from build123d import *

# Parameters (mm, degrees)
SKETCH1_W           = 165.1
SKETCH1_H           = 127
BOSS_EXTRUDE1_DEPTH = 6.35
SKETCH2_W           = 165.1
SKETCH2_H           = 31.75
BOSS_EXTRUDE2_DEPTH = 31.75
CUT_EXTRUDE1_REACH  = 167.1
SKETCH3_R           = 9.525


with BuildPart() as part:
    # Sketch1 → Boss-Extrude1 (new body, symmetric)
    with BuildSketch(Plane(origin=(0, 0, 0), x_dir=(1, 0, 0), z_dir=(0, 1, 0))):
        Rectangle(SKETCH1_W, SKETCH1_H)
    extrude(amount=BOSS_EXTRUDE1_DEPTH, both=True)

    # Sketch2 → Boss-Extrude2 (add)
    with BuildSketch(Plane.XZ.offset(6.35)):
        Rectangle(SKETCH2_W, SKETCH2_H)
    extrude(amount=BOSS_EXTRUDE2_DEPTH)

    # Sketch3 → Cut-Extrude1 (cut, up to next)
    with BuildSketch(Plane(origin=(82.55, 0, 0), x_dir=(0, 0, -1), z_dir=(1, 0, 0)), mode=Mode.PRIVATE) as cut_extrude1_sk1:
        with Locations((0, -22.225)):
            Circle(SKETCH3_R)
    cut_extrude1_tool1 = extrude(cut_extrude1_sk1.sketch, amount=-CUT_EXTRUDE1_REACH, mode=Mode.PRIVATE) & part.part
    add(cut_extrude1_tool1.solids().sort_by_distance((82.55, -22.225, 0))[0], mode=Mode.SUBTRACT)


solid = part.part
The model under review builds one solid part; all positions refer to its coordinate system, in mm. A direction names the side the tool comes from. Round coordinates to 2 decimals unless told otherwise and drop trailing zeros. Order: outer loops, then holes, each group sorted by start corner. A loop starts at its lowest first (then second) coordinate and runs counter-clockwise, first axis right, second up. Notation, with made-up numbers: (34.5, -10.5) - (56.5, -10.5) arc R29 ccw to (56.5, 15.5) - close; hole circle Ø10 at (-34, 52.5). An arc over 180 degrees is marked (long way). Use one line per item in the form item = value.
Q1. Add section D-D on z = -44. Give the boundary of the cut face in (x, y), then the cut area to 3 significant figures.
Response values:
outline = (-82.55, -6.35) - (82.55, -6.35) - (82.55, 6.35) - (-82.55, 6.35) - close
area = 2,100 mm^2
Q2. Add section B-B on y = -24.5. Give the boundary of the cut face in (x, z) (3 decimals), then the cut area to 3 significant figures.
Response values:
outline = (-82.55, -15.875) - (82.55, -15.875) - (82.55, -9.249) - (-82.55, -9.249) - close; (-82.55, 9.249) - (82.55, 9.249) - (82.55, 15.875) - (-82.55, 15.875) - close
area = 2,190 mm^2
Q3. To check wall thickness, follow line 1 (Y direction, x = 41, z = 0); line 2 (Y direction, x = 2.5, z = 43); line 3 (Z direction, x = -41, y = -19) (3 decimals). State the ranges of each line that lie inside material, in increasing order.
Response values:
line_1 = -38.1 to -31.75, -12.7 to 6.35
line_2 = -6.35 to 6.35
line_3 = -15.875 to -8.962, 8.962 to 15.875
Q4. Tool access review of faces 1 (the flat face through (-1, -22, -15.875)), 2 (the flat face through (-1, -22, 15.875)), 3 (the flat face through (82.55, -11, 1)): name each direction out of +Z, -Z, +X, -X, +Y, -Y from which nothing blocks a thin tool from reaching the whole face with its end or side.
Response values:
face_1 = -Z, +X, -X, -Y
face_2 = +Z, +X, -X, -Y
face_3 = +Z, -Z, +X, +Y, -Y
Q5. Mouldability with a two-part tool opening along Y and no side actions: class faces 4 (the flat face through (-82.55, -11, 1)), 5 (the cylindrical face through (1.16, -12.78, 1.24)), 6 (the flat face through (-1, -6.35, 39)) as pulls with the +Y half, pulls with the -Y half, needs draft (parallel to the pull), parting line crosses it, or undercut.
Response values:
face_4 = needs draft
face_5 = undercut
face_6 = pulls with the -Y half
Q6. Clearance check with flat-ended pins moving along their axes: P1, Ø12, axis at y = -15.5, z = 31, coming from the -X side; P2, Ø16, axis at x = -30.5, y = -26, coming from the +Z side (3 decimals); P3, Ø4, axis at x = -30.5, z = 37.5, coming from the -Y side; P4, Ø8, axis at x = -57.5, y = -26, coming from the -Z side (3 decimals). State where each tip first meets the part, or that it passes through.
Response values:
P1 = through
P2 = 15.875
P3 = -6.35
P4 = -15.875
Q7. Add section C-C on x = 36.5. Give the boundary of the cut face in (y, z) (3 decimals), then the cut area to 3 significant figures.
Response values:
outline = (-38.1, -15.875) - (-6.35, -15.875) - (-6.35, -63.5) - (6.35, -63.5) - (6.35, 63.5) - (-6.35, 63.5) - (-6.35, 15.875) - (-38.1, 15.875) - close; hole circle Ø19.05 at (-22.225, 0)
area = 2,340 mm^2
Q8. Add section A-A on z = 0. Give the boundary of the cut face in (x, y).
Response values:
outline = (-82.55, -38.1) - (82.55, -38.1) - (82.55, -31.75) - (-82.55, -31.75) - close; (-82.55, -12.7) - (82.55, -12.7) - (82.55, 6.35) - (-82.55, 6.35) - close
